from build123d import *

# Parameters (mm, degrees)
SKETCH_1_W          = 48
SKETCH_1_H          = 16.97
SKETCH_1_R          = 2.6
EXTRUDE_1_DEPTH     = 10
SKETCH_3_R          = 2.4
CUT_EXTRUDE_1_DEPTH = 6
CUT_EXTRUDE_START   = -6
SKETCH_4_R          = 2.4
CUT_EXTRUDE_2_DEPTH = 6
CUT_EXTRUDE_3_DEPTH = 28.349501367


with BuildPart() as part:
    # ｽｹｯﾁ1 → ﾎﾞｽ - 押し出し1 (new body)
    with BuildSketch(Plane.XY):
        Rectangle(SKETCH_1_W, SKETCH_1_H)
        Circle(SKETCH_1_R, mode=Mode.SUBTRACT)
    extrude(amount=EXTRUDE_1_DEPTH)

    # ｽｹｯﾁ3 → ｶｯﾄ - 押し出し1 (cut)
    with BuildSketch(Plane(origin=(24, 0, 0), x_dir=(0, 0, -1), z_dir=(1, 0, 0))):
        with Locations((-5, 0)):
            Circle(SKETCH_3_R)
    extrude(amount=-CUT_EXTRUDE_1_DEPTH, mode=Mode.SUBTRACT)

    # ｽｹｯﾁ4 → ｶｯﾄ - 押し出し2 (cut)
    with BuildSketch(Plane.ZY.offset(24).offset(CUT_EXTRUDE_START)):
        with Locations(Location((5, 0, 0), (0, 0, 180))):
            Circle(SKETCH_4_R)
    extrude(amount=CUT_EXTRUDE_2_DEPTH, mode=Mode.SUBTRACT)

    # ｽｹｯﾁ5 → ｶｯﾄ - 押し出し3 (cut, through all)
    with BuildSketch(Plane.XY.offset(10)):
        Polygon((-14, 4.985), (14, 4.985), (19, 8.485), (-19, 8.485), align=None)
        Polygon((-14, -4.985), (14, -4.985), (19, -8.485), (-19, -8.485), align=None)
    extrude(amount=-CUT_EXTRUDE_3_DEPTH, mode=Mode.SUBTRACT)


solid = part.part
Part model, mm, in its own coordinate system. A direction names the side the tool comes from. Give positions to 0.01 mm unless a question says otherwise; leave off trailing zeros. Write each loop counter-clockwise with the first axis right and the second up, starting at its lowest first coordinate (ties: lowest second). Pieces come first, ordered by that corner, then holes.
1) Cut at D-D on y = 5.5. Write the cut outline in (x, z), then the cut area to 3 significant figures.
Resolved:
outline: (-24, 0) - (-14.74, 0) - (-14.74, 10) - (-24, 10) - close; (14.74, 0) - (24, 0) - (24, 10) - (14.74, 10) - close
area: 185 mm2
2) Cut at C-C on z = 5. Write the cut outline in (x, y) (3 decimals).
Resolved:
outline: (-24, -8.485) - (-19, -8.485) - (-14, -4.985) - (14, -4.985) - (19, -8.485) - (24, -8.485) - (24, -2.4) - (18, -2.4) - (18, 2.4) - (24, 2.4) - (24, 8.485) - (19, 8.485) - (14, 4.985) - (-14, 4.985) - (-19, 8.485) - (-24, 8.485) - (-24, 2.4) - (-18, 2.4) - (-18, -2.4) - (-24, -2.4) - close; hole circle Ø5.2 at (0, 0)
3) Cut at B-B on y = 0. Write the cut outline in (x, z).
Resolved:
outline: (-24, 0) - (-2.6, 0) - (-2.6, 10) - (-24, 10) - (-24, 7.4) - (-18, 7.4) - (-18, 2.6) - (-24, 2.6) - close; (2.6, 0) - (24, 0) - (24, 2.6) - (18, 2.6) - (18, 7.4) - (24, 7.4) - (24, 10) - (2.6, 10) - close
4) Pin check, flat tips, straight feed: pin 1 (1.4 mm diameter, centred on y = -0.5, z = 5.5, fed in from +X); pin 2 (3 mm diameter, centred on x = 4, z = 2.5, fed in from +Y) (3 decimals); pin 3 (3 mm diameter, centred on y = 0, z = 5, fed in from -X). Stop position of each tip, or through.
Resolved:
pin 1: stops at x = 18
pin 2: stops at y = 4.985
pin 3: stops at x = -18
5) Probe L1, parallel to Y at x = -22.45, z = 5 (3 decimals); L2, parallel to X at y = 1, z = 6; L3, parallel to Y at x = 0, z = 2.5 (3 decimals). List the from-to ranges inside material, lowest first.
Resolved:
L1: y = -8.485 to -2.4, 2.4 to 8.485
L2: x = -18 to -2.4, 2.4 to 18
L3: y = -4.985 to -2.6, 2.6 to 4.985
6) Cut at A-A on x = -1. Write the cut outline in (y, z) (3 decimals), then the cut area to 3 significant figures.
Resolved:
outline: (-4.985, 0) - (-2.4, 0) - (-2.4, 10) - (-4.985, 10) - close; (2.4, 0) - (4.985, 0) - (4.985, 10) - (2.4, 10) - close
area: 51.7 mm2
7) Two-plate mould, pull along Z, no slides. Class faces 1 (the face through (-22, 8.485, 5)), 2 (the face through (0, 4, 0)), 3 (the face through (-20.96, -0.72, 2.71)): released by +Z, released by -Z, zero draft, split by the parting line, or undercut.
Resolved:
face 1: zero draft
face 2: released by -Z
face 3: undercut
8) Which spindle directions (+Z, -Z, +X, -X, +Y, -Y) get a long thin tool onto all of the face, cutting with end or side? Do faces 4 (the face through (16.465, -6.711, 5.07)), 5 (the face through (16.465, 6.711, 5.07)), 6 (the face through (24, 2, 3)), 7 (the face through (18, 0, 5)), 8 (the face through (-18, 0, 5)). Say none if no direction does.
Resolved:
face 4: +Z, -Z, -Y
face 5: +Z, -Z, +Y
face 6: +Z, -Z, +X, +Y, -Y
face 7: +X
face 8: -X
